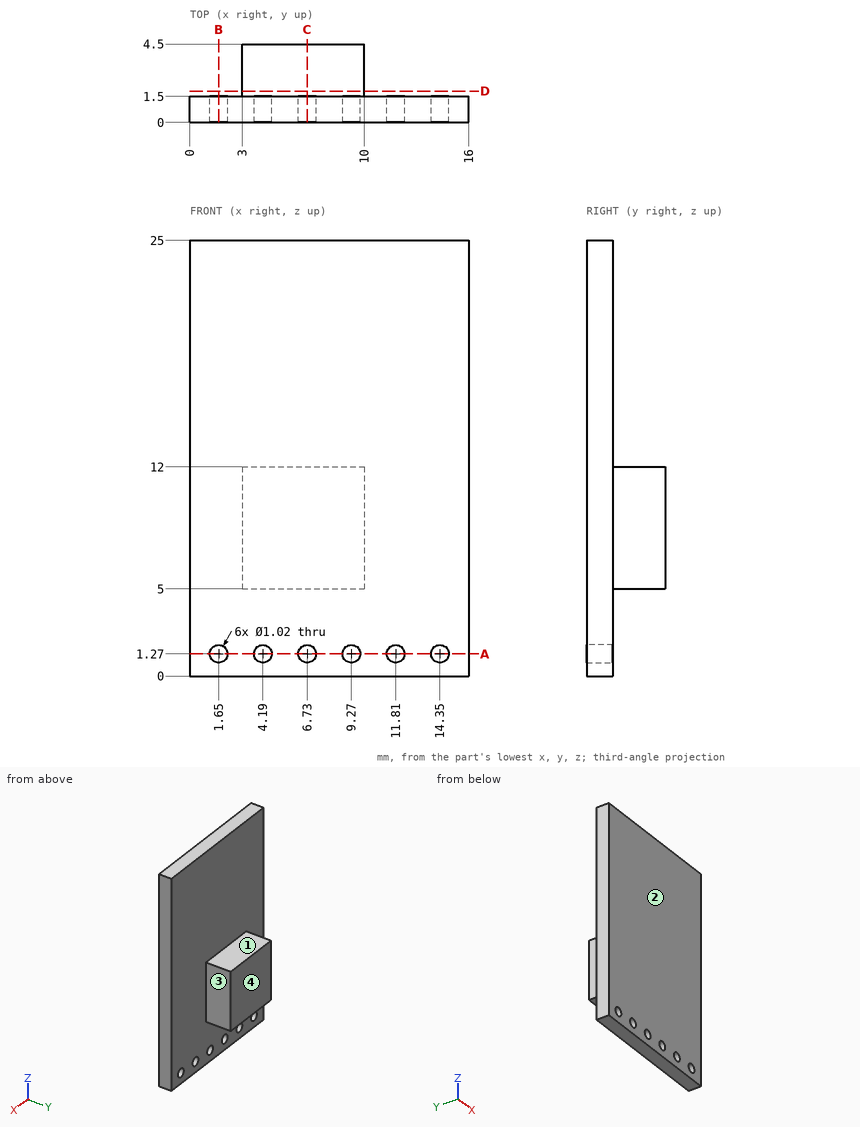
Here's the drawing with two shaded views (mm, measured from the low corner). I have some questions. A direction names the side the tool comes from. Coordinates: 2 decimals unless noted, no trailing zeros. Order: outer loops, then holes, each group sorted by start corner. A loop starts at its lowest first (then second) coordinate and runs counter-clockwise, first axis right, second up. Notation, with made-up numbers: (46, 70) - (94, 70) arc R25 ccw to (94, 108) - close; hole circle Ø1 at (46, 2.5). An arc over 180 degrees is marked (long way). Answer in a Markdown table with one row per item.
1. For pin 1 (0.9 mm diameter, centred on y = 3.5, z = 9, fed in from +X); pin 2 (5 mm diameter, centred on x = 9.5, z = 18.5, fed in from +Y); pin 3 (0.8 mm diameter, centred on x = 14.35, z = 1.27, fed in from +Y); pin 4 (2.5 mm diameter, centred on y = 3, z = 8.5, fed in from -X), each with a flat end and sliding along its axis, tell me the tip position at first contact or that it passes through.
Reply:
| item | result |
|---|---|
| pin 1 | stops at x = 10 |
| pin 2 | stops at y = 1.5 |
| pin 3 | passes through |
| pin 4 | stops at x = 3 |
2. Suppose I cut it at A-A (z = 1.27). Please give me the cut outline in (x, y), and give its area (3 significant figures).
Reply:
| item | result |
|---|---|
| outline | (0, 0) - (1.14, 0) - (1.14, 1.5) - (0, 1.5) - close; (2.16, 0) - (3.68, 0) - (3.68, 1.5) - (2.16, 1.5) - close; (4.7, 0) - (6.22, 0) - (6.22, 1.5) - (4.7, 1.5) - close; (7.24, 0) - (8.76, 0) - (8.76, 1.5) - (7.24, 1.5) - close; (9.78, 0) - (11.3, 0) - (11.3, 1.5) - (9.78, 1.5) - close; (12.32, 0) - (13.84, 0) - (13.84, 1.5) - (12.32, 1.5) - close; (14.86, 0) - (16, 0) - (16, 1.5) - (14.86, 1.5) - close |
| area | 14.8 mm^2 |
3. Suppose I cut it at C-C (x = 6.73). Please give me the cut outline in (y, z), and give its area (3 significant figures).
Reply:
| item | result |
|---|---|
| outline | (0, 0) - (1.5, 0) - (1.5, 0.76) - (0, 0.76) - close; (0, 1.78) - (1.5, 1.78) - (1.5, 5) - (4.5, 5) - (4.5, 12) - (1.5, 12) - (1.5, 25) - (0, 25) - close |
| area | 57.0 mm^2 |
4. If I drill on line 1 along Y through (x, z) = (14.25, 22); line 2 along Z through (x, y) = (6.75, 0.75); line 3 along Z through (x, y) = (9.25, 3.2), over which ranges is the centre line in solid material (lowest first)?
Reply:
| item | result |
|---|---|
| line 1 | y = 0 to 1.5 |
| line 2 | z = 0 to 0.76, 1.78 to 25 |
| line 3 | z = 5 to 12 |
5. Suppose I cut it at D-D (y = 1.8). Please give me the cut outline in (x, z), and give its area (3 significant figures).
Reply:
| item | result |
|---|---|
| outline | (3, 5) - (10, 5) - (10, 12) - (3, 12) - close |
| area | 49.0 mm^2 |
6. Suppose I cut it at B-B (x = 1.65). Please give me the cut outline in (y, z).
Reply:
| item | result |
|---|---|
| outline | (0, 0) - (1.5, 0) - (1.5, 0.76) - (0, 0.76) - close; (0, 1.78) - (1.5, 1.78) - (1.5, 25) - (0, 25) - close |
7. For the marked faces 3 and 4, which set-ups out of +Z, -Z, +X, -X, +Y, -Y let a thin tool reach every point of the face, with its end or its side?
Reply:
| item | result |
|---|---|
| face 3 | +Z, -Z, +X, +Y |
| face 4 | +Z, -Z, +X, -X, +Y |
8. If we mould it in two halves opening along Z, with no side actions, what happens to the marked faces 1 and 2? For each: pulls with the +Z half, pulls with the -Z half, needs draft (parallel to the pull), parting line crosses it, or undercut.
Reply:
| item | result |
|---|---|
| face 1 | pulls with the +Z half |
| face 2 | needs draft |
